Work out the finished part from the listing and answer in its coordinate system (mm). A direction names the side the tool comes from. Round coordinates to 2 decimals unless told otherwise and drop trailing zeros. Loops run counter-clockwise (first coordinate to the right, second up) from the corner with the lowest first, then second, coordinate; pieces in that order, holes last. Notation, with made-up numbers: (-39, 20.5) - (-31, 20.5) arc R21 cw to (-31, 26.5) - close; hole circle Ø5 at (-35, -3.5). An arc over 180 degrees is marked (long way). Answer as CSV lines item,"result". Start each with the question number.
Q1. For faces 4 (the face through (9.25, -27, 0)), 5 (the face through (8.76, -57.46, 0.16)), 6 (the face through (24.25, -27, 10)), determine the directions among +Z, -Z, +X, -X, +Y, -Y from which every point of the face is accessible in a straight line to the end or side of a thin tool.
Q2. Section A-A on x = -20.5 is taken. Write down the section's boundary in (y, z), then the cut area to 3 significant figures.
Q3. Straight lines are drawn through the part: L1, parallel to X at y = -12, z = -0.5; L2, parallel to Z at x = 10.5, y = -29.5. For each, find the intervals that lie inside material, in ascending order. Write a range as [from, to].
Q4. The mould has two halves that part along Z. Classify faces 1 (the face through (-24.25, -27, -10)), 2 (the face through (0, -30, -15)), 3 (the face through (-9.25, -27, 0)): +Z half, -Z half, draft (parallel to the pull), parting line (faces both ways), or undercut.
Q5. Section C-C on y = -40 is taken. Write down the section's boundary in (x, z), then the cut area to 3 significant figures.
Q6. Section B-B on z = 9.5 is taken. Write down the section's boundary in (x, y).
Q7. Section D-D on z = -1.5 is taken. Write down the section's boundary in (x, y).
```python
from build123d import *

# Parameters (mm, degrees)
F1_DEPTH = 60
F3_SIZE2 = 5
F3_SIZE  = 1


# Not quite as in the source:
# - a feature names something its author has since deleted; it is built from what else it names


with BuildPart() as f1:
    # F0 (on Front) → F1 (new body)
    with BuildSketch(Plane.XZ):
        Polygon((-9.5, 15), (-24.25, 15), (-24.25, 9.9166666667), (-17.3952847075, 7.6317615692), (-9.5, 10.2635231383), align=None)
        Polygon((-17.3952847075, 7.6317615692), (-24.25, 9.9166666667), (-24.25, 5.3468564717), align=None)
        Polygon((0, 15), (-9.25, 15), (-9.25, 10.3468564717), (-9.25, 4.9166666667), (-9.25, -10.3468564717), (-9.25, -15), (0, -15), align=None)
        Polygon((-9.25, 15), (-9.5, 15), (-9.5, 10.2635231383), (-9.25, 10.3468564717), align=None)
        Polygon((-17.3952847075, -7.6317615692), (-24.25, -9.9166666667), (-24.25, -15), (-9.5, -15), (-9.5, -10.2635231383), align=None)
        Polygon((-24.25, -5.3468564717), (-24.25, -9.9166666667), (-17.3952847075, -7.6317615692), align=None)
        Polygon((-9.25, -10.3468564717), (-9.5, -10.2635231383), (-9.5, -15), (-9.25, -15), align=None)
    extrude(amount=F1_DEPTH)

    # F2: F1 across face


with BuildPart() as f1_1:
    add(f1.part)
    add(f1.part.mirror(Plane(origin=(0, -30, 0), x_dir=(0, 1, 0), z_dir=(1, 0, 0))))

    # F3
    f3_edges = [f1_1.edges().sort_by_distance(p)[0] for p in [
        (-24.25, -60, 10.173428),
        (9.25, -60, 0),
        (16.75, -60, 7.846856),
        (24.25, -60, 10.173428),
        (-16.75, -60, 7.846856),
        (-9.25, -60, 0),
        (-16.75, -60, -7.846856),
        (-24.25, -60, -10.173428),
        (16.75, -60, -7.846856),
        (24.25, -60, -10.173428),
    ]]
    f3_side = f1_1.faces().sort_by_distance((0, -60, 0))[0]
    chamfer(f3_edges, length=F3_SIZE, length2=F3_SIZE2, reference=f3_side)


solid = f1_1.part
```
Findings:
1,face 4,"+Y, -Y"
1,face 5,"-Y"
1,face 6,"+Z, -Z, +X, +Y, -Y"
2,outline,"(-60, -15) - (0, -15) - (0, -6.6) - (-55, -6.6) - (-60, -7.65) - close; (-60, 7.65) - (-55, 6.6) - (0, 6.6) - (0, 15) - (-60, 15) - close"
2,area,"1,000 mm^2"
3,L1,"x = [-9.25, 9.25]"
3,L2,"z = [-15, -9.93], [9.93, 15]"
4,face 1,"draft"
4,face 2,"-Z half"
4,face 3,"undercut"
5,outline,"(-24.25, -15) - (24.25, -15) - (24.25, -5.35) - (9.25, -10.35) - (9.25, 10.35) - (24.25, 5.35) - (24.25, 15) - (-24.25, 15) - (-24.25, 5.35) - (-9.25, 10.35) - (-9.25, -10.35) - (-24.25, -5.35) - close"
5,area,"984 mm^2"
6,outline,"(-24.25, -55) - (-23.25, -60) - (-14.95, -60) - (-11.79, -55) - (-11.79, 0) - (-24.25, 0) - close; (-9.25, -55) - (-8.25, -60) - (8.25, -60) - (9.25, -55) - (9.25, 0) - (-9.25, 0) - close; (11.79, -55) - (14.95, -60) - (23.25, -60) - (24.25, -55) - (24.25, 0) - (11.79, 0) - close"
7,outline,"(-9.25, -55) - (-8.25, -60) - (8.25, -60) - (9.25, -55) - (9.25, 0) - (-9.25, 0) - close"
